The model under review builds one solid part; all positions refer to its coordinate system, in mm. Coordinates: 2 decimals unless noted, no trailing zeros. Loops run counter-clockwise (first coordinate to the right, second up) from the corner with the lowest first, then second, coordinate; pieces in that order, holes last. Notation, with made-up numbers: M 49,81.5 L 99,81.5 A8 cw 99,92.5 Z; hole C -15,0.5 d9. An arc over 180 degrees is marked long. One line per item, written item: value.
```python
from build123d import *

# Parameters (mm, degrees)
F0_W      = 190.5
F0_H      = 190.5
F0_R      = 3.175
F1_DEPTH  = 6.35
F3_DEPTH  = 6.351
F5_DEPTH  = 6.351
F6_R      = 3.175
F6_R_2    = 19.05
F7_DEPTH  = 6.351
F8_R      = 12.7
F9_R      = 6.35
F9_R_2    = 12.7
F10_DEPTH = 6.351
F11_R     = 12.7
F12_DEPTH = 6.351
F13_R     = 5.715
F13_R_2   = 6.35
F14_DEPTH = 6.351


with BuildPart() as f1:
    # F0 (on Top) → F1 (new body)
    with BuildSketch(Plane.XY):
        Rectangle(F0_W, F0_H)
        with Locations((-82.55, -82.55)):
            Circle(F0_R, mode=Mode.SUBTRACT)
        with Locations((82.55, -82.55)):
            Circle(F0_R, mode=Mode.SUBTRACT)
        with Locations((-82.55, 82.55)):
            Circle(F0_R, mode=Mode.SUBTRACT)
        with Locations((82.55, 82.55)):
            Circle(F0_R, mode=Mode.SUBTRACT)
    extrude(amount=F1_DEPTH)

    # F2 (on face) → F3 (cut, through all)
    with BuildSketch(Plane.XY.offset(6.35)):
        with BuildLine():
            Line((57.15, 47.4726), (57.15, 49.53))
            Line((57.15, 49.53), (59.2074, 49.53))
            ThreePointArc((59.2074, 49.53), (55.695199, 50.984801), (57.15, 47.4726))
        make_face()
        with BuildLine():
            Line((59.2074, 49.53), (57.15, 49.53))
            Line((57.15, 49.53), (57.15, 47.4726))
            ThreePointArc((57.15, 47.4726), (58.604801, 48.075199), (59.2074, 49.53))
        make_face()
        with BuildLine():
            Line((88.9, 49.53), (86.8426, 49.53))
            ThreePointArc((86.8426, 49.53), (87.445199, 48.075199), (88.9, 47.4726))
            Line((88.9, 47.4726), (88.9, 49.53))
        make_face()
        with BuildLine():
            ThreePointArc((90.9574, 49.53), (88.9, 51.5874), (86.8426, 49.53))
            Line((86.8426, 49.53), (88.9, 49.53))
            Line((88.9, 49.53), (88.9, 47.4726))
            ThreePointArc((88.9, 47.4726), (90.354801, 48.075199), (90.9574, 49.53))
        make_face()
        with BuildLine():
            ThreePointArc((59.2074, 11.43), (58.604801, 12.884801), (57.15, 13.4874))
            Line((57.15, 13.4874), (57.15, 11.43))
            Line((57.15, 11.43), (59.2074, 11.43))
        make_face()
        with BuildLine():
            Line((57.15, 11.43), (57.15, 13.4874))
            ThreePointArc((57.15, 13.4874), (55.695199, 9.975199), (59.2074, 11.43))
            Line((59.2074, 11.43), (57.15, 11.43))
        make_face()
        with BuildLine():
            Line((88.9, 11.43), (88.9, 13.4874))
            ThreePointArc((88.9, 13.4874), (87.445199, 12.884801), (86.8426, 11.43))
            Line((86.8426, 11.43), (88.9, 11.43))
        make_face()
        with BuildLine():
            ThreePointArc((90.9574, 11.43), (90.354801, 12.884801), (88.9, 13.4874))
            Line((88.9, 13.4874), (88.9, 11.43))
            Line((88.9, 11.43), (86.8426, 11.43))
            ThreePointArc((86.8426, 11.43), (88.9, 9.3726), (90.9574, 11.43))
        make_face()
    extrude(amount=-F3_DEPTH, mode=Mode.SUBTRACT)

    # F4 (on face) → F5 (cut, through all)
    with BuildSketch(Plane.XY.offset(6.35)):
        with BuildLine():
            Line((-44.45, -42.3926), (-44.45, -44.45))
            Line((-44.45, -44.45), (-42.3926, -44.45))
            ThreePointArc((-42.3926, -44.45), (-42.995199, -42.995199), (-44.45, -42.3926))
        make_face()
        with BuildLine():
            Line((-42.3926, -44.45), (-44.45, -44.45))
            Line((-44.45, -44.45), (-44.45, -42.3926))
            ThreePointArc((-44.45, -42.3926), (-45.904801, -45.904801), (-42.3926, -44.45))
        make_face()
        with BuildLine():
            ThreePointArc((44.45, -42.3926), (42.995199, -42.995199), (42.3926, -44.45))
            Line((42.3926, -44.45), (44.45, -44.45))
            Line((44.45, -44.45), (44.45, -42.3926))
        make_face()
        with BuildLine():
            Line((44.45, -44.45), (42.3926, -44.45))
            ThreePointArc((42.3926, -44.45), (44.45, -46.5074), (46.5074, -44.45))
            ThreePointArc((46.5074, -44.45), (45.904801, -42.995199), (44.45, -42.3926))
            Line((44.45, -42.3926), (44.45, -44.45))
        make_face()
        with BuildLine():
            ThreePointArc((-42.3926, 44.45), (-45.904801, 45.904801), (-44.45, 42.3926))
            Line((-44.45, 42.3926), (-44.45, 44.45))
            Line((-44.45, 44.45), (-42.3926, 44.45))
        make_face()
        with BuildLine():
            Line((-44.45, 44.45), (-44.45, 42.3926))
            ThreePointArc((-44.45, 42.3926), (-42.995199, 42.995199), (-42.3926, 44.45))
            Line((-42.3926, 44.45), (-44.45, 44.45))
        make_face()
        with BuildLine():
            ThreePointArc((42.3926, 44.45), (42.995199, 42.995199), (44.45, 42.3926))
            Line((44.45, 42.3926), (44.45, 44.45))
            Line((44.45, 44.45), (42.3926, 44.45))
        make_face()
        with BuildLine():
            Line((44.45, 44.45), (44.45, 42.3926))
            ThreePointArc((44.45, 42.3926), (45.904801, 42.995199), (46.5074, 44.45))
            ThreePointArc((46.5074, 44.45), (44.45, 46.5074), (42.3926, 44.45))
            Line((42.3926, 44.45), (44.45, 44.45))
        make_face()
    extrude(amount=-F5_DEPTH, mode=Mode.SUBTRACT)

    # F6 (on face) → F7 (cut, through all)
    with BuildSketch(Plane.XY.offset(6.35)):
        with Locations((-33.3375, -34.925)):
            Circle(F6_R)
        with Locations((33.3375, -34.925)):
            Circle(F6_R)
        with Locations((0, 32.385)):
            Circle(F6_R)
        Circle(F6_R_2)
    extrude(amount=-F7_DEPTH, mode=Mode.SUBTRACT)

    # F8
    f8_edges = [f1.edges().sort_by_distance(p)[0] for p in [
        (-95.25, 95.25, 3.175),
        (95.25, 95.25, 3.175),
        (95.25, -95.25, 3.175),
        (-95.25, -95.25, 3.175),
    ]]
    fillet(f8_edges, radius=F8_R)

    # F9 (on face) → F10 (cut, through all)
    with BuildSketch(Plane.XY.offset(6.35)):
        with Locations((62.410512, 62.410512)):
            Circle(F9_R)
        with Locations((0, 69.85)):
            Circle(F9_R_2)
        with Locations((-62.410512, 62.410512)):
            Circle(F9_R)
        with Locations((69.85, 0)):
            Circle(F9_R)
        with Locations((-69.85, 0)):
            Circle(F9_R)
    extrude(amount=-F10_DEPTH, mode=Mode.SUBTRACT)

    # F11 (on face) → F12 (cut, through all)
    with BuildSketch(Plane.XY.offset(6.35)):
        with Locations((-69.85, -33.928976)):
            Circle(F11_R)
        with Locations((-33.928976, -69.85)):
            Circle(F11_R)
        with Locations((69.85, -33.928976)):
            Circle(F11_R)
        with Locations((33.928976, -69.85)):
            Circle(F11_R)
    extrude(amount=-F12_DEPTH, mode=Mode.SUBTRACT)

    # F13 (on face) → F14 (cut, through all)
    with BuildSketch(Plane.XY.offset(6.35)):
        with Locations((-76.2, 35.56)):
            Circle(F13_R)
        with Locations((-38.1, 79.375)):
            Circle(F13_R_2)
        with Locations((38.1, 79.375)):
            Circle(F13_R_2)
        with Locations((0, -76.2)):
            Circle(F13_R_2)
    extrude(amount=-F14_DEPTH, mode=Mode.SUBTRACT)


solid = f1.part
```
(1) Add section A-A on x = 0. State the section outline as (y, z) points.
Checks:
outline: M -95.25,0 L -82.55,0 L -82.55,6.35 L -95.25,6.35 Z; M -69.85,0 L -19.05,0 L -19.05,6.35 L -69.85,6.35 Z; M 19.05,0 L 29.21,0 L 29.21,6.35 L 19.05,6.35 Z; M 35.56,0 L 57.15,0 L 57.15,6.35 L 35.56,6.35 Z; M 82.55,0 L 95.25,0 L 95.25,6.35 L 82.55,6.35 Z
(2) Add section C-C on x = 39. State the section outline as (y, z) points, then the cut area to 3 significant figures.
Checks:
outline: M -95.25,0 L -81.49,0 L -81.49,6.35 L -95.25,6.35 Z; M -58.21,0 L 73.09,0 L 73.09,6.35 L -58.21,6.35 Z; M 85.66,0 L 95.25,0 L 95.25,6.35 L 85.66,6.35 Z
area: 982 mm^2
(3) Insertion check: pin 1 Ø14.5 at (x, y) = (0, -76.2) entering from +Z. The pin has a flat end and moves straight along its axis. Give the tip position at first contact, or say it passes through.
Checks:
pin 1: z = 6.35
(4) Add section B-B on y = 0. State the section outline as (x, z) points.
Checks:
outline: M -95.25,0 L -76.2,0 L -76.2,6.35 L -95.25,6.35 Z; M -63.5,0 L -19.05,0 L -19.05,6.35 L -63.5,6.35 Z; M 19.05,0 L 63.5,0 L 63.5,6.35 L 19.05,6.35 Z; M 76.2,0 L 95.25,0 L 95.25,6.35 L 76.2,6.35 Z
(5) Draft analysis for pull direction X (two halves, no side actions). For faces 1 (the face through (-95.25, -1, 3)), 2 (the face through (-1, 95.25, 3)), 3 (the face through (84.015, 79.733, 3.131)), state which applies: pulls with the +X half, pulls with the -X half, needs draft (parallel to the pull), parting line crosses it, or undercut.
Checks:
face 1: pulls with the -X half
face 2: needs draft
face 3: undercut
(6) Add section D-D on z = 4.5. State how many separate pieces and enclosed holes the cut face has, then the cut area to 3 significant figures.
Checks:
separate pieces: 1
enclosed holes: 29
area: 31,200 mm^2
(7) To check wall thickness, follow L1, parallel to Y at x = -69.85, z = 4; L2, parallel to X at y = 49.53, z = 1.75; L3, parallel to X at y = -22.5, z = 2. State the ranges of each line that lie inside material, in increasing order. Write a range as [from, to].
Checks:
L1: [-95.25, -46.63], [-21.23, -6.35], [6.35, 95.25]
L2: [-95.25, 55.09], [59.21, 86.84], [90.96, 95.25]
L3: [-95.25, -75.39], [-64.31, 64.31], [75.39, 95.25]
